Work out the finished part from the listing and answer in its coordinate system (mm). A direction names the side the tool comes from. Give positions to 0.01 mm unless a question says otherwise; leave off trailing zeros. Loops run counter-clockwise (first coordinate to the right, second up) from the corner with the lowest first, then second, coordinate; pieces in that order, holes last. Notation, with made-up numbers: M 20.25,-25.5 L 28.25,-25.5 A21 ccw 28.25,-14.5 Z; hole C 69.25,65.5 d1. An arc over 180 degrees is marked long. Use a Markdown table: item, result.
```python
from build123d import *

# Parameters (mm, degrees)
SKETCH1_W                      = 26
SKETCH1_H                      = 20
M3X0_5_TAPPED_HOLE1_D          = 2.5
M3X0_5_TAPPED_HOLE1_DEPTH      = 6
M3X0_5_TAPPED_HOLE1_TIP        = 0.751075774
HOLE1_D                        = 25.4
HOLE1_CBORE_D                  = 40
HOLE1_CBORE_DEPTH              = 3.4
M4X0_7_TAPPED_HOLE1_D          = 3.3
M4X0_7_TAPPED_HOLE2_D          = 3.3
M4X0_7_TAPPED_HOLE2_DEPTH      = 13.407641206
F_4_CLEARANCE_HOLE3_D          = 3.3
CBORE_FOR_M3_SHCS1_D           = 3.6
CBORE_FOR_M3_SHCS1_CBORE_D     = 6.5
CBORE_FOR_M3_SHCS1_CBORE_DEPTH = 7.5


with BuildPart() as part:
    # Sketch1 → Revolve1 (revolve)
    with BuildSketch(Plane.XZ, mode=Mode.PRIVATE) as revolve1_sk:
        with Locations((13, 10)):
            Rectangle(SKETCH1_W, SKETCH1_H)
    revolve(revolve1_sk.sketch.rotate(Axis((0, 0, 20), (0, 0, -1)), 180), axis=Axis((0, 0, 20), (0, 0, -1)))

    # M3x0.5 Tapped Hole1
    with Locations(Plane(origin=(0, 0, 0), x_dir=(-1, 0, 0), z_dir=(0, 0, -1))):
        with Locations((-22.776165581, 3.200981322)):
            Hole(M3X0_5_TAPPED_HOLE1_D / 2, depth=M3X0_5_TAPPED_HOLE1_DEPTH)
            with Locations((0, 0, -(M3X0_5_TAPPED_HOLE1_DEPTH + M3X0_5_TAPPED_HOLE1_TIP / 2))):  # 118° drill point
                Cone(0, M3X0_5_TAPPED_HOLE1_D / 2, M3X0_5_TAPPED_HOLE1_TIP, mode=Mode.SUBTRACT)

    # Hole1 (through all)
    with Locations(Plane(origin=(0, 0, 0), x_dir=(-1, 0, 0), z_dir=(0, 0, -1))):
        with Locations((0, 0)):
            CounterBoreHole(HOLE1_D / 2, HOLE1_CBORE_D / 2, HOLE1_CBORE_DEPTH)

    # M4x0.7 Tapped Hole1 (through all)
    with Locations(Plane(origin=(26, 0, 10), x_dir=(0, 1, 0), z_dir=(1, 0, 0))):
        with Locations((0, 0)):
            Hole(M4X0_7_TAPPED_HOLE1_D / 2)

    # M4x0.7 Tapped Hole2
    with Locations(Plane(origin=(0, 12.592358794, 0), x_dir=(-1, 0, 0), z_dir=(0, -1, 0))):
        with Locations((0, -10)):
            Hole(M4X0_7_TAPPED_HOLE2_D / 2, depth=M4X0_7_TAPPED_HOLE2_DEPTH)

    # #4 Clearance Hole3 (through all)
    with Locations(Plane(origin=(0, -12.592358794, 0), x_dir=(1, 0, 0), z_dir=(0, 1, 0))):
        with Locations((0, -10)):
            Hole(F_4_CLEARANCE_HOLE3_D / 2)

    # CBORE for M3 SHCS1 (through all)
    with Locations(Plane(origin=(0, 0, 0), x_dir=(-1, 0, 0), z_dir=(0, 0, -1))):
        with Locations((-15.5, -15.5), (-15.5, 15.5), (15.5, 15.5), (15.5, -15.5)):
            CounterBoreHole(CBORE_FOR_M3_SHCS1_D / 2, CBORE_FOR_M3_SHCS1_CBORE_D / 2, CBORE_FOR_M3_SHCS1_CBORE_DEPTH)


solid = part.part
```
(1) Which of the six approach directions +Z, -Z, +X, -X, +Y, -Y give full straight-line access (tool end or side, diameter ignored) to faces 5 (the flat face through (8, -19, 0)), 6 (the cylindrical face through (-17.25, 18.24, 3.7))?
Entries:
| item | result |
|---|---|
| face 5 | -Z, +X, -X, +Y, -Y |
| face 6 | -Z |
(2) Consider probe 1 along X at (y, z) = (-14, 14); probe 2 along X at (y, z) = (-16.5, 3.75); probe 3 along Y at (x, z) = (-15.5, 5.75). Determine where each line is inside the solid, lowest interval first. Write a range as [from, to].
Entries:
| item | result |
|---|---|
| probe 1 | x = [-21.91, -16.49], [-14.51, 14.51], [16.49, 21.91] |
| probe 2 | x = [-20.09, -18.59], [-12.41, 12.41], [18.59, 20.09] |
| probe 3 | y = [-20.87, -18.75], [-12.25, 12.25], [18.75, 20.87] |
(3) The mould has two halves that part along Z. Classify faces 1 (the flat face through (-17, -17, 7.5)), 2 (the cylindrical face through (-19.4, 0.4, 8.4)), 3 (the cylindrical face through (-20, 0, 2)), 4 (the cylindrical face through (0.4, -19.4, 11.6)): released by +Z, released by -Z, zero draft, split by the parting line, or undercut.
Entries:
| item | result |
|---|---|
| face 1 | released by -Z |
| face 2 | undercut |
| face 3 | zero draft |
| face 4 | undercut |
(4) Given P1, Ø2, axis at y = -18, z = 17, coming from the -X side; P2, Ø5, axis at x = 15.5, y = -15.5, coming from the -Z side; P3, Ø1.5, axis at x = 22.78, y = 3.2, coming from the -Z side, each flat-ended and moving along its own axis, determine where each tip first touches the part or whether it passes through.
Entries:
| item | result |
|---|---|
| P1 | stops at x = -19.67 |
| P2 | stops at z = 7.5 |
| P3 | stops at z = 6.3 |
(5) A cutting plane is placed at B-B (y = 0). Write down the section's boundary in (x, z).
Entries:
| item | result |
|---|---|
| outline | M -26,0 L -20,0 L -20,3.4 L -12.7,3.4 L -12.7,8.35 L -26,8.35 Z; M -26,11.65 L -12.7,11.65 L -12.7,20 L -26,20 Z; M 12.7,3.4 L 20,3.4 L 20,0 L 26,0 L 26,8.35 L 12.7,8.35 Z; M 12.7,11.65 L 26,11.65 L 26,20 L 12.7,20 Z |
(6) A cutting plane is placed at A-A (z = 10). Write down the section's boundary in (x, y).
Entries:
| item | result |
|---|---|
| outline | M -25.95,-1.65 A26 ccw -1.65,-25.95 L -1.65,-12.59 A12.7 cw -12.59,-1.65 Z; M -25.95,1.65 L -12.59,1.65 A12.7 cw -1.65,12.59 L -1.65,25.95 A26 ccw Z; M 1.65,-25.95 A26 ccw 25.95,-1.65 L 12.59,-1.65 A12.7 cw 1.65,-12.59 Z; M 1.65,12.59 A12.7 cw 12.59,1.65 L 25.95,1.65 A26 ccw 1.65,25.95 Z; hole C -15.5,-15.5 d3.6; hole C -15.5,15.5 d3.6; hole C 15.5,-15.5 d3.6; hole C 15.5,15.5 d3.6 |
(7) A cutting plane is placed at D-D (x = -9). Write down the section's boundary in (y, z), and give its area (3 significant figures).
Entries:
| item | result |
|---|---|
| outline | M -24.39,0 L -17.86,0 L -17.86,3.4 L -8.96,3.4 L -8.96,20 L -24.39,20 Z; M 8.96,3.4 L 17.86,3.4 L 17.86,0 L 24.39,0 L 24.39,20 L 8.96,20 Z |
| area | 557 mm² |
